Verification items for the finished model (mm, model axes). A direction names the side the tool comes from. Round coordinates to 2 decimals unless told otherwise and drop trailing zeros. Order: outer loops, then holes, each group sorted by start corner. A loop starts at its lowest first (then second) coordinate and runs counter-clockwise, first axis right, second up. Notation, with made-up numbers: (-7.5, 65.25) -> (35.5, 65.25) arc R19 cw to (35.5, 71.25) -> close; hole circle Ø5 at (-14.5, 16.25). An arc over 180 degrees is marked (long way). Return JSON: item names as keys, results as strings. Group by question number.
Item 1: Sectioned sample at B-B on x = -2.25. Record the cut outline in (y, z).
Item 2: Scan lines: probe 1 along X at (y, z) = (7.8, 1.2); probe 2 along X at (y, z) = (8.25, 11); probe 3 along Y at (x, z) = (-4.75, 16). Record each from-to range of solid material in increasing order. Write a range as from..to.
Item 3: Sectioned sample at A-A on z = 35.5. Record the cut outline in (x, y), plus the area to 3 significant figures.
Item 4: Access from +Z, -Z, +X, -X, +Y, -Y to the whole of each face (thin tool, end or side, straight path). Record for faces 4 (the flat face through (-1, 7, 45.4)), 5 (the flat face through (-11.5, 1.5, 23.5)), 6 (the flat face through (-11.5, 0.8, 20.5)).
Item 5: Draft check along X on faces 1 (the cylindrical face through (-1.8, 7, 0.8)), 2 (the flat face through (-12, 1, 24)), 3 (the flat face through (-11.5, 0.8, 26.5)). Enter one of: pulls with the +X half, pulls with the -X half, needs draft (parallel to the pull), parting line crosses it, or undercut.
Item 6: Depth check by flat-ended pin: pin 1 Ø6 at (x, z) = (-10.5, 22.5) entering from -Y; pin 2 Ø0.8 at (x, y) = (-11.5, 1) entering from -Z; pin 3 Ø5 at (y, z) = (6, 28.5) entering from -X; pin 4 Ø5 at (y, z) = (3.5, 31.5) entering from +X. Enter the tip coordinate at first touch or a pass-through.
Item 7: Sectioned sample at C-C on y = 2.25. Record the cut outline in (x, z), plus the area to 3 significant figures.
Item 8: Sectioned sample at D-D on x = -7. Record the cut outline in (y, z).
```python
from build123d import *

# Parameters (mm, degrees)
F1_DEPTH = 47
F2_W     = 8.6
F2_H     = 43.8
F3_DEPTH = 25
F4_D     = 1
F5_W     = 1.5
F5_H     = 6
F6_DEPTH = 1


with BuildPart() as f1:
    # F0 (on Top) → F1 (new body)
    with BuildSketch(Plane.XY):
        with BuildLine():
            ThreePointArc((-2.891366459, 8.6), (-1.8165902125, 7.0125327227), (0, 6.4))
            Line((0, 6.4), (0, 8.15))
            ThreePointArc((0, 8.15), (-0.0211310131, 8.3788689869), (-0.083809621, 8.6))
            Line((-0.083809621, 8.6), (-2.891366459, 8.6))
        make_face()
        with BuildLine():
            Line((-10.2, 9.4), (-10.2, 8.6))
            Line((-10.2, 8.6), (-2.891366459, 8.6))
            Line((-2.891366459, 8.6), (-0.083809621, 8.6))
            ThreePointArc((-0.083809621, 8.6), (-0.5428932188, 9.1807764064), (-1.25, 9.4))
            Line((-1.25, 9.4), (-10.2, 9.4))
        make_face()
        Polygon((-11, 0), (-10.2, 0), (-10.2, 8.6), (-10.2, 9.4), (-11, 9.4), align=None)
    extrude(amount=F1_DEPTH)

    # F2 (on face) → F3 (cut)
    with BuildSketch(Plane.YZ.offset(-10.2)):
        with Locations((4.3, 23.5)):
            Rectangle(F2_W, F2_H)
    extrude(amount=F3_DEPTH, mode=Mode.SUBTRACT)

    # F4 (through all)
    with Locations(Plane(origin=(0, 0, 0), x_dir=(1, 0, 0), z_dir=(0, 0, -1))):
        with Locations((-1, -7.8)):
            Hole(F4_D / 2)

    # F5 (on face) → F6 (join)
    with BuildSketch(Plane(origin=(-11, 0, 0), x_dir=(0, -1, 0), z_dir=(-1, 0, 0))):
        with Locations((-0.75, 23.5)):
            Rectangle(F5_W, F5_H)
    extrude(amount=F6_DEPTH)


solid = f1.part
```
Recorded:
{
 "1": {"outline": "(7.42, 0) -> (9.4, 0) -> (9.4, 47) -> (7.42, 47) -> (7.42, 45.4) -> (8.6, 45.4) -> (8.6, 1.6) -> (7.42, 1.6) -> close"},
 "2": {"probe 1": "-11..-10.2, -2.54..-1.5, -0.5..0", "probe 2": "-11..-10.2", "probe 3": "8.6..9.4"},
 "3": {"outline": "(-11, 0) -> (-10.2, 0) -> (-10.2, 8.6) -> (-0.08, 8.6) arc R1.25 ccw to (-1.25, 9.4) -> (-11, 9.4) -> close", "area": "15.4 mm²"},
 "4": {"face 4": "+X, -Y", "face 5": "+Z, -Z, -X, +Y", "face 6": "-Z, -X, +Y, -Y"},
 "5": {"face 1": "undercut", "face 2": "pulls with the -X half", "face 3": "needs draft"},
 "6": {"pin 1": "y = 0", "pin 2": "z = 20.5", "pin 3": "x = -11", "pin 4": "x = -10.2"},
 "7": {"outline": "(-11, 0) -> (-10.2, 0) -> (-10.2, 47) -> (-11, 47) -> close", "area": "37.6 mm²"},
 "8": {"outline": "(8.6, 0) -> (9.4, 0) -> (9.4, 47) -> (8.6, 47) -> close"}
}
